```python
from build123d import *

# Parameters (mm, degrees)
F0_W     = 46
F0_H     = 80
F1_DEPTH = 5
F2_W     = 34
F2_H     = 66
F3_DEPTH = 1
F4_R     = 3
F5_DEPTH = 3
F6_R     = 1.6
F7_DEPTH = 6.001


with BuildPart() as f1:
    # F0 (on Top) → F1 (new body)
    with BuildSketch(Plane.XY):
        with Locations((-1.260705, 0.965576)):
            Rectangle(F0_W, F0_H)
    extrude(amount=F1_DEPTH)

    # F2 (on face) → F3 (join)
    with BuildSketch(Plane.XY.offset(5)):
        with Locations((-1.260705, 0.965576)):
            Rectangle(F2_W, F2_H)
    extrude(amount=F3_DEPTH)

    # F4 (on face) → F5 (cut)
    with BuildSketch(Plane.XY.offset(6)):
        with Locations((-19.337287, 28.25648)):
            Circle(F4_R)
        with Locations((16.662713, 28.25648)):
            Circle(F4_R)
        with Locations((-19.337287, -27.74352)):
            Circle(F4_R)
        with Locations((16.662713, -27.74352)):
            Circle(F4_R)
    extrude(amount=-F5_DEPTH, mode=Mode.SUBTRACT)

    # F6 (on face) → F7 (cut, through all)
    with BuildSketch(Plane.XY.offset(6)):
        with Locations((-19.337287, 28.25648)):
            Circle(F6_R)
        with Locations((16.662713, 28.25648)):
            Circle(F6_R)
        with Locations((-19.337287, -27.74352)):
            Circle(F6_R)
        with Locations((16.662713, -27.74352)):
            Circle(F6_R)
    extrude(amount=-F7_DEPTH, mode=Mode.SUBTRACT)


solid = f1.part
```
Work out the finished part from the listing and answer in its coordinate system (mm). A direction names the side the tool comes from. Give positions to 0.01 mm unless a question says otherwise; leave off trailing zeros. Write each loop counter-clockwise with the first axis right and the second up, starting at its lowest first coordinate (ties: lowest second). Pieces come first, ordered by that corner, then holes. Notation, with made-up numbers: (20, 70.25) - (36, 70.25) arc R18 cw to (36, 95.25) - close; hole circle Ø1 at (6, 71.25). An arc over 180 degrees is marked (long way). Use one line per item in the form item = value.
1. A cutting plane is placed at B-B (y = 18). Write down the section's boundary in (x, z), and give its area (3 significant figures).
Filled in:
outline = (-24.26, 0) - (21.74, 0) - (21.74, 5) - (15.74, 5) - (15.74, 6) - (-18.26, 6) - (-18.26, 5) - (-24.26, 5) - close
area = 264 mm^2
2. Each of these flat-tipped pins is pushed along its axis until it touches: pin 1 Ø0.5 at (y, z) = (0.5, 5.5) entering from -X; pin 2 Ø6.5 at (x, y) = (-20.5, 28) entering from +Z; pin 3 Ø3.5 at (x, y) = (-19.34, 28.26) entering from +Z; pin 4 Ø1.9 at (x, y) = (-19.34, -27.74) entering from -Z. Where does it stop, or does it pass through?
Filled in:
pin_1 = -18.26
pin_2 = 5
pin_3 = 3
pin_4 = through
3. A cutting plane is placed at A-A (x = 2). Write down the section's boundary in (y, z).
Filled in:
outline = (-39.03, 0) - (40.97, 0) - (40.97, 5) - (33.97, 5) - (33.97, 6) - (-32.03, 6) - (-32.03, 5) - (-39.03, 5) - close
4. Consider L1, parallel to Y at x = -19, z = 3.6; L2, parallel to Y at x = 16.5, z = 4.9; L3, parallel to X at y = 27.5, z = 2.15. Determine where each line is inside the solid, lowest interval first.
Filled in:
L1 = -39.03 to -30.72, -24.76 to 25.28, 31.24 to 40.97
L2 = -39.03 to -30.74, -24.75 to 25.26, 31.25 to 40.97
L3 = -24.26 to -20.75, -17.93 to 15.25, 18.07 to 21.74
5. Determine the mould class of faces 3 (the face through (18, -29, 3)), 4 (the face through (-2, 40.966, 2)), 5 (the face through (-1, 1, 6)), 6 (the face through (-18, 27, 3)) for opening direction Y: released by +Y, released by -Y, zero draft, split by the parting line, or undercut.
Filled in:
face_3 = undercut
face_4 = released by +Y
face_5 = zero draft
face_6 = undercut
6. For faces 1 (the face through (21.739, 0, 2)), 2 (the face through (13.666, 28.388, 4.188)), determine the directions among +Z, -Z, +X, -X, +Y, -Y from which every point of the face is accessible in a straight line to the end or side of a thin tool.
Filled in:
face_1 = +Z, -Z, +X, +Y, -Y
face_2 = +Z
